Work out the finished part from the listing and answer in its coordinate system (mm). A direction names the side the tool comes from. Coordinates: 2 decimals unless noted, no trailing zeros. Order: outer loops, then holes, each group sorted by start corner. A loop starts at its lowest first (then second) coordinate and runs counter-clockwise, first axis right, second up. Notation, with made-up numbers: M 48,1.25 L 106,1.25 A18 cw 106,12.25 Z; hole C -26.75,65 d11. An arc over 180 degrees is marked long. Use a Markdown table: item, result. Add a question column.
from build123d import *

# Parameters (mm, degrees)
F0_W     = 130
F0_H     = 296
F1_DEPTH = 10
F2_SIZE2 = 29.99999
F2_SIZE  = 19.99999
F3_SIZE2 = 19.99999
F3_SIZE  = 49.99999
F4_T     = 2.5


# Not quite as in the source:
# - a fillet or chamfer is up to 0.001 mm smaller than in the source, because OpenCascade refuses the exact size
# - a shell that OpenCascade refuses in one call is made with other operations: the cavity is built on its own and cut out


with BuildPart() as f1:
    # F0 (on Top) → F1 (new body, symmetric)
    with BuildSketch(Plane.XY):
        Rectangle(F0_W, F0_H)
    extrude(amount=F1_DEPTH, both=True)

    # F2 (size 20 and 30 in the source; OpenCascade refuses exactly that, so slightly less here)
    f2_edges = [f1.edges().sort_by_distance(p)[0] for p in [
        (0, -148, -10),
    ]]
    f2_side = f1.faces().sort_by_distance((0, -148, 0))[0]
    chamfer(f2_edges, length=F2_SIZE, length2=F2_SIZE2, reference=f2_side)

    # F3 (size 50 and 20 in the source; OpenCascade refuses exactly that, so slightly less here)
    f3_edges = [f1.edges().sort_by_distance(p)[0] for p in [
        (0, 148, -10),
    ]]
    f3_side = f1.faces().sort_by_distance((0, 14.999995, -10))[0]
    chamfer(f3_edges, length=F3_SIZE, length2=F3_SIZE2, reference=f3_side)

    # F4: shell of thickness 2.5, made by hand


with BuildPart() as f4_core1:
    # F4_t2: copy of F1
    add(f1.part)

    # the walls: a layer under each face that stays
    f4_faces = [f4_core1.faces().sort_by_distance(p)[0] for p in [
        (65, 0, 0),
        (0, -10, -10),
        (0, 123.000005, -5e-06),
        (0, -133.000005, -5e-06),
        (0, 148, 9.999995),
        (0, -148, 9.999995),
        (-65, 0, 0),
    ]]
    thicken(f4_faces, amount=-F4_T, mode=Mode.SUBTRACT)


with BuildPart() as f1_1:
    add(f1.part)

    # what is left inside the walls is the cavity
    f4_cavity = [f4_core1.part.solids().sort_by_distance(p)[0] for p in [
        (0, -48.572528, 9.975),
    ]]
    add(f4_cavity, mode=Mode.SUBTRACT)


solid = f1_1.part
(1) A cutting plane is placed at B-B on y = 32.5. Write down the section's boundary in (x, z), plus the area to 4 significant figures.
(2) A cutting plane is placed at A-A on z = 4. Write down the section's boundary in (x, y), plus the area to 3 significant figures.
(3) The mould has two halves that part along Y. Classify faces 1 (the flat face through (62.5, -3, 1)), 2 (the flat face through (-1, 123, 0)), 3 (the flat face through (65, -2, 0)): pulls with the +Y half, pulls with the -Y half, needs draft (parallel to the pull), parting line crosses it, or undercut.
(4) A cutting plane is placed at D-D on y = 104.5. Write down the section's boundary in (x, z).
(5) Which of the six approach directions +Z, -Z, +X, -X, +Y, -Y give full straight-line access (tool end or side, diameter ignored) to faces 4 (the flat face through (-0.875, 119.7, 1.372)), 5 (the flat face through (-1, -8, -10))?
(6) Given P1, Ø3, axis at x = 47.5, z = 5, coming from the -Y side; P2, Ø1.5, axis at x = 26.5, z = 5, coming from the -Y side (3 decimals); P3, Ø1, axis at x = 19.5, z = 0.5, coming from the -Y side, each flat-ended and moving along its own axis, determine where each tip first touches the part or whether it passes through.
(7) Straight lines are drawn through the part: line 1 (X direction, y = 72, z = 0.75); line 2 (Z direction, x = 40.5, y = -6); line 3 (Z direction, x = -49, y = 131). For each, find the intervals that lie inside material, in ascending order.
From the geometry:
| question | item | result |
|---|---|---|
| 1 | outline | M -65,-10 L 65,-10 L 65,10 L 62.5,10 L 62.5,-7.5 L -62.5,-7.5 L -62.5,10 L -65,10 Z |
| 1 | area | 412.5 mm2 |
| 2 | outline | M -65,-139 L 65,-139 L 65,133 L -65,133 Z; hole M -62.5,-134.49 L 62.5,-134.49 L 62.5,126.27 L -62.5,126.27 Z |
| 2 | area | 2,760 mm2 |
| 3 | face 1 | undercut |
| 3 | face 2 | pulls with the +Y half |
| 3 | face 3 | needs draft |
| 4 | outline | M -65,-7.4 L 65,-7.4 L 65,10 L 62.5,10 L 62.5,-4.71 L -62.5,-4.71 L -62.5,10 L -65,10 Z |
| 5 | face 4 | +Z |
| 5 | face 5 | -Z, +X, -X, +Y, -Y |
| 6 | P1 | stops at y = -142.75 |
| 6 | P2 | stops at y = -141.625 |
| 6 | P3 | stops at y = -134.5 |
| 7 | line 1 | x = -65 to -62.5, 62.5 to 65 |
| 7 | line 2 | z = -10 to -7.5 |
| 7 | line 3 | z = 3.2 to 5.89 |
